Autodesk Inventor part; units mm, degrees
ref_plane "YZ Plane" through (0, 0, 0) normal (1, 0, 0) x (0, 1, 0)
ref_plane "XZ Plane" through (0, 0, 0) normal (0, 1, 0) x (-1, 0, 0)
ref_plane "XY Plane" through (0, 0, 0) normal (0, 0, 1) x (1, 0, 0)
sketch "Sketch1" plane through (0, 0, 0) normal (0, 1, 0) x (-1, 0, 0)
  circle A0 centre (0, 0) radius 1.755
  circle A1 centre (0, 0) radius 1.475
  dimension "d0" = 3.51
  dimension "d1" = 2.95
extrude "Extrusion1" add sketch "Sketch1" along normal blind 100
sketch "Sketch2" plane through (0, 100, 0) normal (0, 1, 0) x (1, 0, 0)
  circle A0 centre (0, 0) radius 1.755
  circle A1 centre (0, 0) radius 1.475
  circle A2 centre (0, 0) radius 6.755
  dimension "d4" = 5
extrude "Extrusion2" add sketch "Sketch2" along normal blind 0.3 contours A0 | A2
sketch "Sketch3" plane through (0, 100.3, 0) normal (0, 1, 0) x (1, 0, 0)
  circle A0 centre (0, 0) radius 1.755
  circle A1 centre (0, 0) radius 1.475
extrude "Extrusion3" add sketch "Sketch3" along normal blind 39
properties part number "Shield"
Model file for the job. Use its own axes, mm. A direction names the side the tool comes from. Give positions to 0.01 mm unless a question says otherwise; leave off trailing zeros. Loops run counter-clockwise (first coordinate to the right, second up) from the corner with the lowest first, then second, coordinate; pieces in that order, holes last.
1) Wall check: line 1 (Z direction, x = 0, y = 36) (3 decimals); line 2 (Y direction, x = 1.75, z = 1.75). Give the ranges that are in metal, low to high.
2) Saw through at D-D (x = 5.25). Write the cut outline in (y, z), plus the area to 3 significant figures.
3) Flat gauge pins, fed straight in: pin 1 Ø4 at (x, y) = (-1.5, 110.5) entering from +Z (3 decimals); pin 2 Ø6 at (x, y) = (-1, 66.5) entering from -Z (3 decimals); pin 3 Ø3 at (x, y) = (-3, 114.5) entering from +Z. Where does each tip first touch, or does it go through?
4) Saw through at B-B (y = 10). Write the cut outline in (x, z) (3 decimals).
5) Tool access for faces 1 (the cylindrical face through (-6.75, 100.15, 0.3)), 2 (the flat face through (1.4, 100.3, 1.4)), 3 (the cylindrical face through (-1.674, 49.3, -0.527)): list every direction of +Z, -Z, +X, -X, +Y, -Y with a clear straight run to the whole face (end or side of a thin tool).
6) Saw through at C-C (z = -3.75). Write the cut outline in (x, y).
Answer block:
1. line 1: z = -1.755 to -1.475, 1.475 to 1.755
1. line 2: y = 100 to 100.3
2. outline: (100, -4.25) - (100.3, -4.25) - (100.3, 4.25) - (100, 4.25) - close
2. area: 2.55 mm2
3. pin 1: stops at z = 1.755
3. pin 2: stops at z = -1.755
3. pin 3: stops at z = 0.91
4. outline: circle Ø3.51 at (0, 0); hole circle Ø2.95 at (0, 0)
5. face 1: +Y, -Y
5. face 2: +Y
5. face 3: -Y
6. outline: (-5.62, 100) - (5.62, 100) - (5.62, 100.3) - (-5.62, 100.3) - close
